Part model, mm, in its own coordinate system. Face numbers are marked on the shaded views. A direction names the side the tool comes from. Round coordinates to 2 decimals unless told otherwise and drop trailing zeros. Order: outer loops, then holes, each group sorted by start corner. A loop starts at its lowest first (then second) coordinate and runs counter-clockwise, first axis right, second up. Notation, with made-up numbers: (-29.5, 24) - (21.5, 24) arc R32 cw to (21.5, 60) - close; hole circle Ø1 at (67.25, 71). An arc over 180 degrees is marked (long way). Return JSON: item names as keys, results as strings. Group by question number.
Item 1: Tool access for the marked faces 4 and 5: list every direction of +Z, -Z, +X, -X, +Y, -Y with a clear straight run to the whole face (end or side of a thin tool).
Item 2: Saw through at A-A on x = -1. List the corners of the cut face in (y, z).
Item 3: Probe probe 1 along Y at (x, z) = (11.5, 5); probe 2 along X at (y, z) = (6.25, 8.5); probe 3 along Z at (x, y) = (12.5, 0.5). List the from-to ranges inside material, lowest first.
Item 4: Two-plate mould, pull along X, no slides. Class the marked faces 1, 2 and 3: released by +X, released by -X, zero draft, split by the parting line, or undercut.
Item 5: Drop flat-ended pins along their axis: pin 1 (21.5 mm diameter, centred on x = -6.5, z = 4, fed in from +Y); pin 2 (8 mm diameter, centred on x = 14, z = 7, fed in from +Y); pin 3 (1 mm diameter, centred on y = 2.5, z = 16, fed in from +X); pin 4 (6 mm diameter, centred on x = 9, z = -9.5, fed in from -Y). Give the stop position or say it passes through.
Item 6: Saw through at D-D on z = -17. List the corners of the cut face in (x, y), and give its area (3 significant figures).
Item 7: Saw through at B-B on z = 0. List the corners of the cut face in (x, y), and give its area (3 significant figures).
Item 8: Saw through at C-C on y = 6.25. List the corners of the cut face in (x, z).
```python
from build123d import *

# Parameters (mm, degrees)
ESQUISSE1_R             = 26.5
BOSS_EXTRU_1_DEPTH      = 8
ESQUISSE2_R             = 21.5
ESQUISSE2_R_2           = 6.75
ENL_V_MAT_EXTRU_1_DEPTH = 6
ESQUISSE3_R             = 2.5
ENL_V_MAT_EXTRU_2_DEPTH = 39.321012513
ESQUISSE4_R             = 5
ENL_V_MAT_EXTRU_3_DEPTH = 38.953919429


with BuildPart() as part:
    # Esquisse1 → Boss.-Extru.1 (new body)
    with BuildSketch(Plane(origin=(0, 0, 0), x_dir=(1, 0, 0), z_dir=(0, 1, 0))):
        with Locations(Location((0, 0, 0), (0, 0, 270))):
            Circle(ESQUISSE1_R)
    extrude(amount=BOSS_EXTRU_1_DEPTH)

    # Esquisse2 → Enlèv. mat.-Extru.1 (cut)
    with BuildSketch(Plane(origin=(0, 8, 0), x_dir=(1, 0, 0), z_dir=(0, 1, 0))):
        with Locations(Location((0, 0, 0), (0, 0, 270))):
            Circle(ESQUISSE2_R)
        with Locations(Location((0, 0, 0), (0, 0, 270))):
            Circle(ESQUISSE2_R_2, mode=Mode.SUBTRACT)
    extrude(amount=-ENL_V_MAT_EXTRU_1_DEPTH, mode=Mode.SUBTRACT)

    # Esquisse3 → Enlèv. mat.-Extru.2 (cut, through all)
    with BuildSketch(Plane(origin=(0, 8, 0), x_dir=(1, 0, 0), z_dir=(0, 1, 0))):
        with Locations(Location((0, 0, 0), (0, 0, 270))):
            Circle(ESQUISSE3_R)
    extrude(amount=-ENL_V_MAT_EXTRU_2_DEPTH, mode=Mode.SUBTRACT)

    # Esquisse4 → Enlèv. mat.-Extru.3 (cut, through all)
    with BuildSketch(Plane(origin=(0, 2, 0), x_dir=(-1, 0, 0), z_dir=(0, 1, 0))):
        with Locations(Location((13.961193072, -2.144927276, 0), (0, 0, 90))):
            Circle(ESQUISSE4_R)
        with Locations(Location((-5.123035026, 13.163211505, 0), (0, 0, 90))):
            Circle(ESQUISSE4_R)
        with Locations(Location((-8.838158046, -11.018284229, 0), (0, 0, 90))):
            Circle(ESQUISSE4_R)
    extrude(amount=-ENL_V_MAT_EXTRU_3_DEPTH, mode=Mode.SUBTRACT)


solid = part.part
```
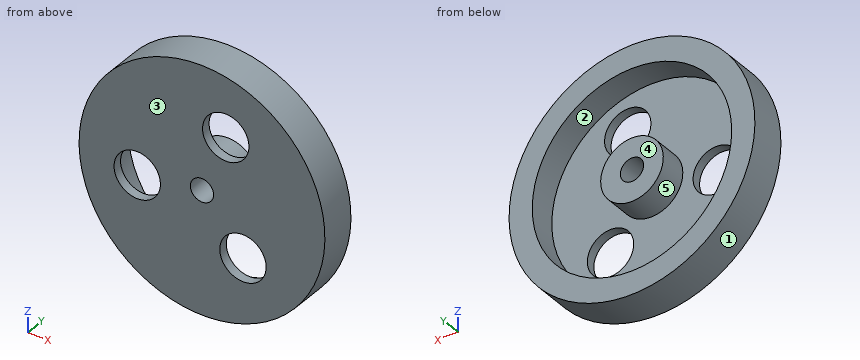
Filled in:
{
 "1": {"face 4": "+Z, -Z, +X, -X, +Y", "face 5": "+Y"},
 "2": {"outline": "(0, -26.48) - (8, -26.48) - (8, -21.48) - (2, -21.48) - (2, -6.68) - (8, -6.68) - (8, -2.29) - (0, -2.29) - close; (0, 2.29) - (8, 2.29) - (8, 6.68) - (2, 6.68) - (2, 21.48) - (8, 21.48) - (8, 26.48) - (0, 26.48) - close"},
 "3": {"probe 1": "y = 0 to 2", "probe 2": "x = -25.1 to -19.75, 19.75 to 25.1", "probe 3": "z = -23.37 to -14.42, -7.61 to 23.37"},
 "4": {"face 1": "split by the parting line", "face 2": "undercut", "face 3": "zero draft"},
 "5": {"pin 1": "stops at y = 8", "pin 2": "stops at y = 2", "pin 3": "stops at x = 21.49", "pin 4": "passes through"},
 "6": {"outline": "(-20.33, 0) - (20.33, 0) - (20.33, 8) - (13.16, 8) - (13.16, 2) - (-13.16, 2) - (-13.16, 8) - (-20.33, 8) - close", "area": "167 mm^2"},
 "7": {"outline": "(-26.5, 0) - (-18.48, 0) - (-18.48, 2) - (-21.5, 2) - (-21.5, 8) - (-26.5, 8) - close; (-9.44, 0) - (-2.5, 0) - (-2.5, 8) - (-6.75, 8) - (-6.75, 2) - (-9.44, 2) - close; (2.5, 0) - (26.5, 0) - (26.5, 8) - (21.5, 8) - (21.5, 2) - (6.75, 2) - (6.75, 8) - (2.5, 8) - close", "area": "189 mm^2"},
 "8": {"outline": "circle Ø53 at (0, 0); circle Ø13.5 at (0, 0); hole circle Ø43 at (0, 0); hole circle Ø5 at (0, 0)"}
}
